Work out the finished part from the listing and answer in its coordinate system (mm). Coordinates: 2 decimals unless noted, no trailing zeros. Answer as a JSON object with one key per item and string values. Group by question number.
1) The mould has two halves that part along X. Classify faces 1 (the face through (33.96, 1.48, -23)), 2 (the face through (-46.317, 1.479, -30.104)), 3 (the face through (-60.93, 1.48, -33.21)), 4 (the face through (46.142, 1.479, -33.135)): released by +X, released by -X, zero draft, split by the parting line, or undercut.
2) This flat-tipped pin is pushed along its axis until it touches: P1, Ø2.5, axis at x = -12.43, z = -23.89, coming from the -Y side. Where does it stop, or does it pass through?
3) Section A-A (z = -24) is taken. Count the separate pieces of the cut face and the enclosed holes in it, plus the area to 3 significant figures.
4) Find the intervals of material crossed by line 1 along Z through (x, y) = (-47.5, 2.35); line 2 along Z through (x, y) = (-3, 2.6); line 3 along X through (y, z) = (0.9, -32.25), in increasing order.
from build123d import *

# Parameters (mm, degrees)
SKETCH1_R           = 1.65
BOSS_EXTRUDE1_DEPTH = 3


with BuildPart() as part:
    # Sketch1 → Boss-Extrude1 (new body)
    with BuildSketch(Plane(origin=(0, 0, 0), x_dir=(1, 0, 0), z_dir=(0, 1, 0))):
        with BuildLine():
            Line((-57.431827558, 14.388379565), (42.568172442, 14.388379565))
            ThreePointArc((42.568172442, 14.388379565), (46.103706348, 15.852845659), (47.568172442, 19.388379565))
            Line((47.568172442, 19.388379565), (47.568172442, 29.638379565))
            ThreePointArc((47.568172442, 29.638379565), (46.103706348, 33.173913471), (42.568172442, 34.638379565))
            Line((42.568172442, 34.638379565), (-57.431827558, 34.638379565))
            ThreePointArc((-57.431827558, 34.638379565), (-60.967361464, 33.173913471), (-62.431827558, 29.638379565))
            Line((-62.431827558, 29.638379565), (-62.431827558, 19.388379565))
            ThreePointArc((-62.431827558, 19.388379565), (-60.967361464, 15.852845659), (-57.431827558, 14.388379565))
        make_face()
        with Locations(Location((-57.431827558, 28.888379565, 0), (0, 0, 270))):
            Circle(SKETCH1_R, mode=Mode.SUBTRACT)
        with Locations(Location((-52.431827558, 28.888379565, 0), (0, 0, 270))):
            Circle(SKETCH1_R, mode=Mode.SUBTRACT)
        with Locations(Location((-47.431827558, 28.888379565, 0), (0, 0, 270))):
            Circle(SKETCH1_R, mode=Mode.SUBTRACT)
        with Locations(Location((-42.431827558, 28.888379565, 0), (0, 0, 270))):
            Circle(SKETCH1_R, mode=Mode.SUBTRACT)
        with Locations(Location((-37.431827558, 28.888379565, 0), (0, 0, 270))):
            Circle(SKETCH1_R, mode=Mode.SUBTRACT)
        with Locations(Location((-32.431827558, 28.888379565, 0), (0, 0, 270))):
            Circle(SKETCH1_R, mode=Mode.SUBTRACT)
        with Locations(Location((-27.431827558, 28.888379565, 0), (0, 0, 270))):
            Circle(SKETCH1_R, mode=Mode.SUBTRACT)
        with Locations(Location((-22.431827558, 28.888379565, 0), (0, 0, 270))):
            Circle(SKETCH1_R, mode=Mode.SUBTRACT)
        with Locations(Location((-17.431827558, 28.888379565, 0), (0, 0, 270))):
            Circle(SKETCH1_R, mode=Mode.SUBTRACT)
        with Locations(Location((-12.431827558, 28.888379565, 0), (0, 0, 270))):
            Circle(SKETCH1_R, mode=Mode.SUBTRACT)
        with Locations(Location((-7.431827558, 28.888379565, 0), (0, 0, 270))):
            Circle(SKETCH1_R, mode=Mode.SUBTRACT)
        with Locations(Location((-2.431827558, 28.888379565, 0), (0, 0, 270))):
            Circle(SKETCH1_R, mode=Mode.SUBTRACT)
        with Locations(Location((2.568172442, 28.888379565, 0), (0, 0, 270))):
            Circle(SKETCH1_R, mode=Mode.SUBTRACT)
        with Locations(Location((7.568172442, 28.888379565, 0), (0, 0, 270))):
            Circle(SKETCH1_R, mode=Mode.SUBTRACT)
        with Locations(Location((12.568172442, 28.888379565, 0), (0, 0, 270))):
            Circle(SKETCH1_R, mode=Mode.SUBTRACT)
        with Locations(Location((17.568172442, 28.888379565, 0), (0, 0, 270))):
            Circle(SKETCH1_R, mode=Mode.SUBTRACT)
        with Locations(Location((22.568172442, 28.888379565, 0), (0, 0, 270))):
            Circle(SKETCH1_R, mode=Mode.SUBTRACT)
        with Locations(Location((27.568172442, 28.888379565, 0), (0, 0, 270))):
            Circle(SKETCH1_R, mode=Mode.SUBTRACT)
        with Locations(Location((32.568172442, 28.888379565, 0), (0, 0, 270))):
            Circle(SKETCH1_R, mode=Mode.SUBTRACT)
        with Locations(Location((37.568172442, 28.888379565, 0), (0, 0, 270))):
            Circle(SKETCH1_R, mode=Mode.SUBTRACT)
        with Locations(Location((42.568172442, 28.888379565, 0), (0, 0, 270))):
            Circle(SKETCH1_R, mode=Mode.SUBTRACT)
        with Locations(Location((-52.431827558, 23.888379565, 0), (0, 0, 270))):
            Circle(SKETCH1_R, mode=Mode.SUBTRACT)
        with Locations(Location((-47.431827558, 23.888379565, 0), (0, 0, 270))):
            Circle(SKETCH1_R, mode=Mode.SUBTRACT)
        with Locations(Location((-42.431827558, 23.888379565, 0), (0, 0, 270))):
            Circle(SKETCH1_R, mode=Mode.SUBTRACT)
        with Locations(Location((-37.431827558, 23.888379565, 0), (0, 0, 270))):
            Circle(SKETCH1_R, mode=Mode.SUBTRACT)
        with Locations(Location((-32.431827558, 23.888379565, 0), (0, 0, 270))):
            Circle(SKETCH1_R, mode=Mode.SUBTRACT)
        with Locations(Location((-27.431827558, 23.888379565, 0), (0, 0, 270))):
            Circle(SKETCH1_R, mode=Mode.SUBTRACT)
        with Locations(Location((-22.431827558, 23.888379565, 0), (0, 0, 270))):
            Circle(SKETCH1_R, mode=Mode.SUBTRACT)
        with Locations(Location((-17.431827558, 23.888379565, 0), (0, 0, 270))):
            Circle(SKETCH1_R, mode=Mode.SUBTRACT)
        with Locations(Location((-12.431827558, 23.888379565, 0), (0, 0, 270))):
            Circle(SKETCH1_R, mode=Mode.SUBTRACT)
        with Locations(Location((-7.431827558, 23.888379565, 0), (0, 0, 270))):
            Circle(SKETCH1_R, mode=Mode.SUBTRACT)
        with Locations(Location((-2.431827558, 23.888379565, 0), (0, 0, 270))):
            Circle(SKETCH1_R, mode=Mode.SUBTRACT)
        with Locations(Location((2.568172442, 23.888379565, 0), (0, 0, 270))):
            Circle(SKETCH1_R, mode=Mode.SUBTRACT)
        with Locations(Location((7.568172442, 23.888379565, 0), (0, 0, 270))):
            Circle(SKETCH1_R, mode=Mode.SUBTRACT)
        with Locations(Location((12.568172442, 23.888379565, 0), (0, 0, 270))):
            Circle(SKETCH1_R, mode=Mode.SUBTRACT)
        with Locations(Location((17.568172442, 23.888379565, 0), (0, 0, 270))):
            Circle(SKETCH1_R, mode=Mode.SUBTRACT)
        with Locations(Location((22.568172442, 23.888379565, 0), (0, 0, 270))):
            Circle(SKETCH1_R, mode=Mode.SUBTRACT)
        with Locations(Location((27.568172442, 23.888379565, 0), (0, 0, 270))):
            Circle(SKETCH1_R, mode=Mode.SUBTRACT)
        with Locations(Location((32.568172442, 23.888379565, 0), (0, 0, 270))):
            Circle(SKETCH1_R, mode=Mode.SUBTRACT)
        with Locations(Location((37.568172442, 23.888379565, 0), (0, 0, 270))):
            Circle(SKETCH1_R, mode=Mode.SUBTRACT)
        with Locations(Location((42.568172442, 23.888379565, 0), (0, 0, 270))):
            Circle(SKETCH1_R, mode=Mode.SUBTRACT)
        with Locations(Location((-57.431827558, 23.888379565, 0), (0, 0, 270))):
            Circle(SKETCH1_R, mode=Mode.SUBTRACT)
    extrude(amount=BOSS_EXTRUDE1_DEPTH)


solid = part.part
Report:
{
 "1": {"face 1": "undercut", "face 2": "undercut", "face 3": "released by -X", "face 4": "released by +X"},
 "2": {"P1": "passes through"},
 "3": {"separate pieces": "22", "enclosed holes": "0", "area": "123 mm²"},
 "4": {"line 1": "z = -34.64 to -30.54, -27.24 to -25.54, -22.24 to -14.39", "line 2": "z = -34.64 to -30.44, -27.34 to -25.44, -22.34 to -14.39", "line 3": "x = -61.7 to 46.83"}
}
